from build123d import *

# Parameters (mm, degrees)
F1_DEPTH = 8


with BuildPart() as f1:
    # F0 (on Front) → F1 (new body)
    with BuildSketch(Plane.XZ):
        Polygon((0, 23.0557063947), (0, 16.8315059189), (5, 16.8315059189), (10.202977498, 30.9157529595), (6.807, 30.9157529595), (6.807, 26.9857296771), align=None)
        Polygon((10.202977498, 30.9157529595), (11.25, 33.75), (0, 45), (0, 38.7757995242), (6.807, 34.8457762418), (6.807, 30.9157529595), align=None)
        Polygon((-5, 16.8315059189), (0, 16.8315059189), (0, 23.0557063947), (-6.807, 26.9857296771), (-6.807, 30.9157529595), (-10.202977498, 30.9157529595), align=None)
        Polygon((0, 45), (-11.25, 33.75), (-10.202977498, 30.9157529595), (-6.807, 30.9157529595), (-6.807, 34.8457762418), (0, 38.7757995242), align=None)
        Polygon((4.9234117813, -16.8315059189), (0, -16.8315059189), (0, -23.0557063947), (6.807, -26.9857296771), (6.807, -30.9157529595), (10.1901471638, -30.9157529595), align=None)
        Polygon((0, -45), (11.25, -33.75), (10.1901471638, -30.9157529595), (6.807, -30.9157529595), (6.807, -34.8457762418), (0, -38.7757995242), align=None)
        Polygon((0, -23.0557063947), (0, -16.8315059189), (-5.2934198313, -16.8315059189), (-10.2521322445, -30.9157529595), (-6.807, -30.9157529595), (-6.807, -26.9857296771), align=None)
        Polygon((-10.2521322445, -30.9157529595), (-11.25, -33.75), (0, -45), (0, -38.7757995242), (-6.807, -34.8457762418), (-6.807, -30.9157529595), align=None)
        Polygon((23.0557063947, 0), (16.8315059189, 0), (16.8315059189, -5), (30.9157529595, -10.202977498), (30.9157529595, -6.807), (26.9857296771, -6.807), align=None)
        Polygon((30.9157529595, -6.807), (30.9157529595, -10.202977498), (33.75, -11.25), (45, 0), (38.7757995242, 0), (34.8457762418, -6.807), align=None)
        Polygon((16.8315059189, 5), (16.8315059189, 0), (23.0557063947, 0), (26.9857296771, 6.807), (30.9157529595, 6.807), (30.9157529595, 10.202977498), align=None)
        Polygon((33.75, 11.25), (30.9157529595, 10.202977498), (30.9157529595, 6.807), (34.8457762418, 6.807), (38.7757995242, 0), (45, 0), align=None)
        Polygon((-23.0557063947, 0), (-16.8315059189, 0), (-16.8315059189, 5), (-30.9157529595, 10.202977498), (-30.9157529595, 6.807), (-26.9857296771, 6.807), align=None)
        Polygon((-30.9157529595, 10.202977498), (-33.75, 11.25), (-45, 0), (-38.7757995242, 0), (-34.8457762418, 6.807), (-30.9157529595, 6.807), align=None)
        Polygon((-16.8315059189, -4.9234117813), (-16.8315059189, 0), (-23.0557063947, 0), (-26.9857296771, -6.807), (-30.9157529595, -6.807), (-30.9157529595, -10.1901471638), align=None)
        Polygon((-45, 0), (-33.75, -11.25), (-30.9157529595, -10.1901471638), (-30.9157529595, -6.807), (-34.8457762418, -6.807), (-38.7757995242, 0), align=None)
        with BuildLine():
            Line((0, -16.8315059189), (0, -13))
            ThreePointArc((0, -13), (-2.7059805904, -12.7152534007), (-5.2934198313, -11.8734875453))
            Line((-5.2934198313, -11.8734875453), (-5.2934198313, -16.8315059189))
            Line((-5.2934198313, -16.8315059189), (0, -16.8315059189))
        make_face()
        with BuildLine():
            ThreePointArc((4.9234117813, -12.031625677), (2.5088708814, -12.7556092328), (0, -13))
            Line((0, -13), (0, -16.8315059189))
            Line((0, -16.8315059189), (4.9234117813, -16.8315059189))
            Line((4.9234117813, -16.8315059189), (4.9234117813, -12.031625677))
        make_face()
        with BuildLine():
            ThreePointArc((4.9234117813, -9.6478773263), (2.5318451875, -10.5314424662), (0, -10.8315059189))
            Line((0, -10.8315059189), (0, -13))
            ThreePointArc((0, -13), (2.5088708814, -12.7556092328), (4.9234117813, -12.031625677))
            Line((4.9234117813, -12.031625677), (4.9234117813, -9.6478773263))
        make_face()
        with BuildLine():
            Line((0, -13), (0, -10.8315059189))
            ThreePointArc((0, -10.8315059189), (-2.7353719229, -10.4804227451), (-5.2934198313, -9.4499326432))
            Line((-5.2934198313, -9.4499326432), (-5.2934198313, -11.8734875453))
            ThreePointArc((-5.2934198313, -11.8734875453), (-2.7059805904, -12.7152534007), (0, -13))
        make_face()
        with BuildLine():
            ThreePointArc((-5.2934198313, -9.4499326432), (-6.5378382821, -8.63586655), (-7.6590312857, -7.6590312857))
            Line((-7.6590312857, -7.6590312857), (-9.1923881554, -9.1923881554))
            ThreePointArc((-9.1923881554, -9.1923881554), (-7.3659168976, -10.7118284274), (-5.2934198313, -11.8734875453))
            Line((-5.2934198313, -11.8734875453), (-5.2934198313, -9.4499326432))
        make_face()
        with BuildLine():
            Line((-9.1923881554, -9.1923881554), (-7.6590312857, -7.6590312857))
            ThreePointArc((-7.6590312857, -7.6590312857), (-8.7608889358, -6.3693284989), (-9.6478773263, -4.9234117813))
            Line((-9.6478773263, -4.9234117813), (-12.031625677, -4.9234117813))
            ThreePointArc((-12.031625677, -4.9234117813), (-10.8245429747, -7.1992547802), (-9.1923881554, -9.1923881554))
        make_face()
        with BuildLine():
            ThreePointArc((-9.6478773263, -4.9234117813), (-10.5314424662, -2.5318451875), (-10.8315059189, 0))
            Line((-10.8315059189, 0), (-13, 0))
            ThreePointArc((-13, 0), (-12.7556092328, -2.5088708814), (-12.031625677, -4.9234117813))
            Line((-12.031625677, -4.9234117813), (-9.6478773263, -4.9234117813))
        make_face()
        with BuildLine():
            ThreePointArc((-12.031625677, -4.9234117813), (-12.7556092328, -2.5088708814), (-13, 0))
            Line((-13, 0), (-16.8315059189, 0))
            Line((-16.8315059189, 0), (-16.8315059189, -4.9234117813))
            Line((-16.8315059189, -4.9234117813), (-12.031625677, -4.9234117813))
        make_face()
        with BuildLine():
            Line((-16.8315059189, 0), (-13, 0))
            ThreePointArc((-13, 0), (-12.747548784, 2.5495097568), (-12, 5))
            Line((-12, 5), (-16.8315059189, 5))
            Line((-16.8315059189, 5), (-16.8315059189, 0))
        make_face()
        with BuildLine():
            Line((-13, 0), (-10.8315059189, 0))
            ThreePointArc((-10.8315059189, 0), (-10.5212893153, 2.5737116418), (-9.6084088418, 5))
            Line((-9.6084088418, 5), (-12, 5))
            ThreePointArc((-12, 5), (-12.747548784, 2.5495097568), (-13, 0))
        make_face()
        with BuildLine():
            ThreePointArc((-9.6084088418, 5), (-8.7354870491, 6.4041226165), (-7.6590312857, 7.6590312857))
            Line((-7.6590312857, 7.6590312857), (-9.1923881554, 9.1923881554))
            ThreePointArc((-9.1923881554, 9.1923881554), (-10.8015442666, 7.2337156051), (-12, 5))
            Line((-12, 5), (-9.6084088418, 5))
        make_face()
        with BuildLine():
            Line((-9.1923881554, 9.1923881554), (-7.6590312857, 7.6590312857))
            ThreePointArc((-7.6590312857, 7.6590312857), (-6.4041226165, 8.7354870491), (-5, 9.6084088418))
            Line((-5, 9.6084088418), (-5, 12))
            ThreePointArc((-5, 12), (-7.2337156051, 10.8015442666), (-9.1923881554, 9.1923881554))
        make_face()
        with BuildLine():
            Line((0, 16.8315059189), (0, 13))
            ThreePointArc((0, 13), (2.5495097568, 12.747548784), (5, 12))
            Line((5, 12), (5, 16.8315059189))
            Line((5, 16.8315059189), (0, 16.8315059189))
        make_face()
        with BuildLine():
            ThreePointArc((-5, 9.6084088418), (-2.5737116418, 10.5212893153), (0, 10.8315059189))
            Line((0, 10.8315059189), (0, 13))
            ThreePointArc((0, 13), (-2.5495097568, 12.747548784), (-5, 12))
            Line((-5, 12), (-5, 9.6084088418))
        make_face()
        with BuildLine():
            Line((0, 13), (0, 10.8315059189))
            ThreePointArc((0, 10.8315059189), (2.5737116418, 10.5212893153), (5, 9.6084088418))
            Line((5, 9.6084088418), (5, 12))
            ThreePointArc((5, 12), (2.5495097568, 12.747548784), (0, 13))
        make_face()
        with BuildLine():
            ThreePointArc((5, 9.6084088418), (6.4041226165, 8.7354870491), (7.6590312857, 7.6590312857))
            Line((7.6590312857, 7.6590312857), (9.1923881554, 9.1923881554))
            ThreePointArc((9.1923881554, 9.1923881554), (7.2337156051, 10.8015442666), (5, 12))
            Line((5, 12), (5, 9.6084088418))
        make_face()
        with BuildLine():
            ThreePointArc((7.6590312857, 7.6590312857), (8.7354870491, 6.4041226165), (9.6084088418, 5))
            Line((9.6084088418, 5), (12, 5))
            ThreePointArc((12, 5), (10.8015442666, 7.2337156051), (9.1923881554, 9.1923881554))
            Line((9.1923881554, 9.1923881554), (7.6590312857, 7.6590312857))
        make_face()
        with BuildLine():
            ThreePointArc((9.6084088418, 5), (10.5212893153, 2.5737116418), (10.8315059189, 0))
            Line((10.8315059189, 0), (13, 0))
            ThreePointArc((13, 0), (12.747548784, 2.5495097568), (12, 5))
            Line((12, 5), (9.6084088418, 5))
        make_face()
        with BuildLine():
            Line((9.1923881554, -9.1923881554), (7.6590312857, -7.6590312857))
            ThreePointArc((7.6590312857, -7.6590312857), (6.3693284989, -8.7608889358), (4.9234117813, -9.6478773263))
            Line((4.9234117813, -9.6478773263), (4.9234117813, -12.031625677))
            ThreePointArc((4.9234117813, -12.031625677), (7.1992547802, -10.8245429747), (9.1923881554, -9.1923881554))
        make_face()
        with BuildLine():
            ThreePointArc((12, 5), (12.747548784, 2.5495097568), (13, 0))
            Line((13, 0), (16.8315059189, 0))
            Line((16.8315059189, 0), (16.8315059189, 5))
            Line((16.8315059189, 5), (12, 5))
        make_face()
        with BuildLine():
            ThreePointArc((-5, 12), (-2.5495097568, 12.747548784), (0, 13))
            Line((0, 13), (0, 16.8315059189))
            Line((0, 16.8315059189), (-5, 16.8315059189))
            Line((-5, 16.8315059189), (-5, 12))
        make_face()
        with BuildLine():
            Line((16.8315059189, 0), (13, 0))
            ThreePointArc((13, 0), (12.747548784, -2.5495097568), (12, -5))
            Line((12, -5), (16.8315059189, -5))
            Line((16.8315059189, -5), (16.8315059189, 0))
        make_face()
        with BuildLine():
            Line((13, 0), (10.8315059189, 0))
            ThreePointArc((10.8315059189, 0), (10.5212893153, -2.5737116418), (9.6084088418, -5))
            Line((9.6084088418, -5), (12, -5))
            ThreePointArc((12, -5), (12.747548784, -2.5495097568), (13, 0))
        make_face()
        with BuildLine():
            Line((12, -5), (9.6084088418, -5))
            ThreePointArc((9.6084088418, -5), (8.7354870491, -6.4041226165), (7.6590312857, -7.6590312857))
            Line((7.6590312857, -7.6590312857), (9.1923881554, -9.1923881554))
            ThreePointArc((9.1923881554, -9.1923881554), (10.8015442666, -7.2337156051), (12, -5))
        make_face()
    extrude(amount=F1_DEPTH)


solid = f1.part
Design review of the part built by this model. Coordinates are the model's own, in mm. A direction names the side the tool comes from. Coordinates: 2 decimals unless noted, no trailing zeros. Order: outer loops, then holes, each group sorted by start corner. A loop starts at its lowest first (then second) coordinate and runs counter-clockwise, first axis right, second up. Notation, with made-up numbers: (23, -11.75) -> (41, -11.75) arc R27 ccw to (41, 22.25) -> close; hole circle Ø6 at (-31.75, 44). An arc over 180 degrees is marked (long way). One line per item, written item: value.
1) We need section D-D, the plane x = 15. Give the boundary of the cut face in (y, z).
Output values:
outline: (-8, -5) -> (0, -5) -> (0, 5) -> (-8, 5) -> close
2) We need section B-B, the plane y = -2.75. Count the separate pieces of the cut face and the enclosed holes in it, then the cut area to 3 significant figures.
Output values:
separate pieces: 1
enclosed holes: 5
area: 1,290 mm2
3) Clearance check with flat-ended pins moving along their axes: P1, Ø1, axis at y = -6, z = -31, coming from the -X side; P2, Ø4, axis at x = 30.5, y = -4.5, coming from the -Z side; P3, Ø1.4, axis at x = 14, y = -5, coming from the +Z side; P4, Ø6, axis at x = 1, z = -35.5, coming from the -Y side. State where each tip first meets the part, or that it passes through.
Output values:
P1: stops at x = -10.46
P2: stops at z = -10.79
P3: stops at z = 5
P4: stops at y = -8
4) We need section A-A, the plane z = -32. Give the boundary of the cut face in (x, y).
Output values:
outline: (-10.63, -8) -> (-6.81, -8) -> (-6.81, 0) -> (-10.63, 0) -> close; (6.81, -8) -> (10.6, -8) -> (10.6, 0) -> (6.81, 0) -> close
5) Draft analysis for pull direction Z (two halves, no side actions). For faces 4 (the face through (39, -4, 6)), 5 (the face through (6, -4, -39)), 6 (the face through (-31, -4, 6.807)), 7 (the face through (-10, 0, 7)), state which applies: +Z half, -Z half, draft (parallel to the pull), parting line (faces both ways), or undercut.
Output values:
face 4: +Z half
face 5: -Z half
face 6: undercut
face 7: draft
6) Machinability: for faces 1 (the face through (24.993, -3.944, 3.356)), 2 (the face through (-5.293, -4, -14)), 3 (the face through (-6, -4, 39)), which of the approach directions +Z, -Z, +X, -X, +Y, -Y give a long, thin tool a straight path to every point of the face, cutting with its end or side? Answer none if there is none.
Output values:
face 1: +Y, -Y
face 2: -X, +Y, -Y
face 3: +Z, -X, +Y, -Y
7) To check wall thickness, follow probe 1 along X at (y, z) = (-4, 1); probe 2 along Z at (x, y) = (2, -3); probe 3 along Z at (x, y) = (3, -0.75). State the ranges of each line that lie inside material, in increasing order. Write a range as [from, to].
Output values:
probe 1: x = [-44, -38.2], [-23.63, -10.79], [10.79, 23.63], [38.2, 44]
probe 2: z = [-43, -37.62], [-24.21, -10.65], [10.65, 24.21], [37.62, 43]
probe 3: z = [-42, -37.04], [-24.79, -10.41], [10.41, 24.79], [37.04, 42]
8) We need section C-C, the plane z = 3. Give the boundary of the cut face in (x, y), then the cut area to 3 significant figures.
Output values:
outline: (-42, -8) -> (-37.04, -8) -> (-37.04, 0) -> (-42, 0) -> close; (-24.79, -8) -> (-10.41, -8) -> (-10.41, 0) -> (-24.79, 0) -> close; (10.41, -8) -> (24.79, -8) -> (24.79, 0) -> (10.41, 0) -> close; (37.04, -8) -> (42, -8) -> (42, 0) -> (37.04, 0) -> close
area: 309 mm2
